Design review of the part built by this model. Coordinates are the model's own, in mm. Face numbers are marked on the shaded views. Give positions to 0.01 mm unless a question says otherwise; leave off trailing zeros. Loops run counter-clockwise (first coordinate to the right, second up) from the corner with the lowest first, then second, coordinate; pieces in that order, holes last. Notation, with made-up numbers: (-7, 80) - (18, 80) arc R25 cw to (18, 117) - close; hole circle Ø4 at (14, 84). An arc over 180 degrees is marked (long way). Write each question's results on one line, items separated by ' | '.
```python
from build123d import *

# Parameters (mm, degrees)
SKETCH_1_W          = 209.4
SKETCH_1_H          = 149.2
EXTRUDE_1_DEPTH     = 7.4
SKETCH_2_W          = 196.3
SKETCH_2_H          = 136
EXTRUDE_2_DEPTH     = 16.5
SKETCH_4_W          = 154.1
SKETCH_4_H          = 85.9
CUT_EXTRUDE_1_DEPTH = 1.5
FILLET_1_R          = 2
SKETCH_5_W          = 199.4
SKETCH_5_H          = 139.2
CUT_EXTRUDE_2_DEPTH = 0.5
FILLET_2_R          = 3


with BuildPart() as part:
    # 草图1 → 凸台-拉伸1 (new body)
    with BuildSketch(Plane.XY):
        Rectangle(SKETCH_1_W, SKETCH_1_H)
    extrude(amount=EXTRUDE_1_DEPTH)

    # 草图2 → 凸台-拉伸2 (add)
    with BuildSketch(Plane.XY.offset(7.4)):
        Rectangle(SKETCH_2_W, SKETCH_2_H)
    extrude(amount=EXTRUDE_2_DEPTH)

    # 草图4 → 切除-拉伸1 (cut)
    with BuildSketch(Plane(origin=(0, 0, 0), x_dir=(-1, 0, 0), z_dir=(0, 0, -1))):
        with Locations((-1.2, 6.2)):
            Rectangle(SKETCH_4_W, SKETCH_4_H)
    extrude(amount=-CUT_EXTRUDE_1_DEPTH, mode=Mode.SUBTRACT)

    # 圆角1
    fillet_1_edges = [part.edges().sort_by_distance(p)[0] for p in [
        (0, 74.6, 0),
        (104.7, 0, 0),
        (0, -74.6, 0),
        (-104.7, 0, 0),
    ]]
    fillet(fillet_1_edges, radius=FILLET_1_R)

    # 草图5 → 切除-拉伸2 (cut)
    with BuildSketch(Plane(origin=(0, 0, 0), x_dir=(-1, 0, 0), z_dir=(0, 0, -1))):
        Rectangle(SKETCH_5_W, SKETCH_5_H)
    extrude(amount=-CUT_EXTRUDE_2_DEPTH, mode=Mode.SUBTRACT)

    # 圆角2
    fillet_2_edges = [part.edges().sort_by_distance(p)[0] for p in [
        (99.7, -69.6, 0.25),
        (99.7, 69.6, 0.25),
        (-99.7, 69.6, 0.25),
        (-99.7, -69.6, 0.25),
    ]]
    fillet(fillet_2_edges, radius=FILLET_2_R)


solid = part.part
```
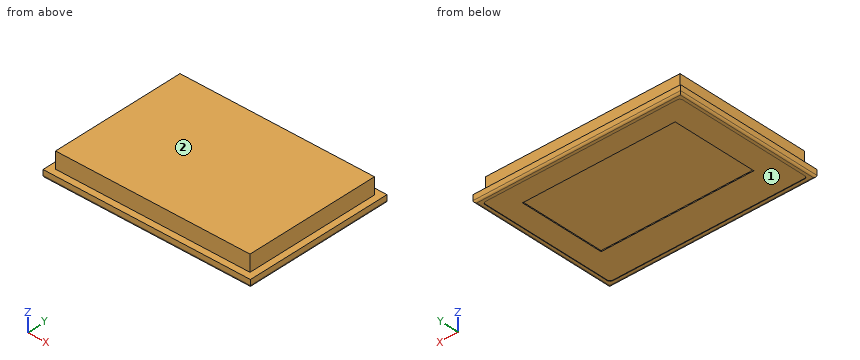
Item 1: We need section B-B on y = -42.5. Give the boundary of the cut face in (x, z).
Output values:
outline: (-104.7, 2) arc R2 ccw to (-102.7, 0) - (-99.7, 0) - (-99.7, 0.5) - (99.7, 0.5) - (99.7, 0) - (102.7, 0) arc R2 ccw to (104.7, 2) - (104.7, 7.4) - (98.15, 7.4) - (98.15, 23.9) - (-98.15, 23.9) - (-98.15, 7.4) - (-104.7, 7.4) - close
Item 2: Wall thickness on probe 1 along X at (y, z) = (-18.5, 15.75); probe 2 along Z at (x, y) = (37.5, -32.5); probe 3 along Z at (x, y) = (85, -22): over which ranges is each line inside the solid? List them lowest first.
Output values:
probe 1: x = -98.15 to 98.15 | probe 2: z = 1.5 to 23.9 | probe 3: z = 0.5 to 23.9
Item 3: We need section C-C on z = 12.25. Give the boundary of the cut face in (x, y), then the cut area to 3 significant figures.
Output values:
outline: (-98.15, -68) - (98.15, -68) - (98.15, 68) - (-98.15, 68) - close | area: 26,700 mm²
Item 4: We need section D-D on y = 17.5. Give the boundary of the cut face in (x, z).
Output values:
outline: (-104.7, 2) arc R2 ccw to (-102.7, 0) - (-99.7, 0) - (-99.7, 0.5) - (-75.85, 0.5) - (-75.85, 1.5) - (78.25, 1.5) - (78.25, 0.5) - (99.7, 0.5) - (99.7, 0) - (102.7, 0) arc R2 ccw to (104.7, 2) - (104.7, 7.4) - (98.15, 7.4) - (98.15, 23.9) - (-98.15, 23.9) - (-98.15, 7.4) - (-104.7, 7.4) - close
Item 5: Clearance check with flat-ended pins moving along their axes: P1, Ø8, axis at x = 42.5, z = 12, coming from the -Y side; P2, Ø1.1, axis at y = 27.5, z = 1, coming from the +X side; P3, Ø5, axis at y = 50.5, z = 14.5, coming from the +X side; P4, Ø12, axis at y = 0.5, z = 9.5, coming from the -X side. State where each tip first meets the part, or that it passes through.
Output values:
P1: stops at y = -68 | P2: stops at x = 104.65 | P3: stops at x = 98.15 | P4: stops at x = -104.7
Item 6: Draft analysis for pull direction Y (two halves, no side actions). For the marked faces 1 and 2, state which applies: +Y half, -Y half, draft (parallel to the pull), parting line (faces both ways), or undercut.
Output values:
face 1: undercut | face 2: draft
Item 7: We need section A-A on x = -78. Give the boundary of the cut face in (y, z), then the cut area to 3 significant figures.
Output values:
outline: (-74.6, 2) arc R2 ccw to (-72.6, 0) - (-69.6, 0) - (-69.6, 0.5) - (69.6, 0.5) - (69.6, 0) - (72.6, 0) arc R2 ccw to (74.6, 2) - (74.6, 7.4) - (68, 7.4) - (68, 23.9) - (-68, 23.9) - (-68, 7.4) - (-74.6, 7.4) - close | area: 3,280 mm²
